Source: CAD feature listing. Evaluate the final solid. Frame: model axes, mm. A direction names the side the tool comes from. Give positions to 0.01 mm unless a question says otherwise; leave off trailing zeros. Loops run counter-clockwise (first coordinate to the right, second up) from the corner with the lowest first, then second, coordinate; pieces in that order, holes last.
from build123d import *

# Parameters (mm, degrees)
BOSS_EXTRUDE1_DEPTH        = 40
SKETCH3_W                  = 100.026130685
SKETCH3_H                  = 60
BOSS_EXTRUDE2_DEPTH        = 25
FILLET1_R                  = 20
F_10_0_10_DIAMETER_HOLE1_D = 10
FILLET1_OF_MIRROR1_R       = 20
DELETEFACE1_START          = -30
DELETEFACE1_DEPTH          = 60
SKETCH16_R                 = 5
BOSS_EXTRUDE3_DEPTH        = 15
RIB1_REACH                 = 138.403
SKETCH18_WALL_W            = 310.161126634
SKETCH18_WALL_H            = 10


# Read off the part's stored shape, not the designer's step: DeleteFace1
with BuildPart() as part:
    # Sketch2 → Boss-Extrude1 (new, symmetric)
    with BuildSketch(Plane.XY):
        with BuildLine():
            Line((-40, 0), (-25, 0))
            ThreePointArc((-25, 0), (0, 25), (25, 0))
            Line((25, 0), (40, 0))
            ThreePointArc((40, 0), (0, 40), (-40, 0))
        make_face()
    extrude(amount=BOSS_EXTRUDE1_DEPTH, both=True)

    # Sketch3 → Boss-Extrude2 (add)
    with BuildSketch(Plane.XZ):
        with Locations((-60.013065343, 0)):
            Rectangle(SKETCH3_W, SKETCH3_H)
    boss_extrude2 = extrude(amount=-BOSS_EXTRUDE2_DEPTH)

    # Fillet1
    fillet1_edges = [part.edges().sort_by_distance(p)[0] for p in [
        (-110.026130685, 12.5, 30),
        (-110.026130685, 12.5, -30),
    ]]
    fillet(fillet1_edges, radius=FILLET1_R)

    # Ø10.0 (10) Diameter Hole1 (through all)
    with Locations(Plane(origin=(0, 25, 0), x_dir=(1, 0, 0), z_dir=(0, 1, 0))):
        with Locations((-90.026130685, -10), (-90.026130685, 11.237902365)):
            f_10_0_10_diameter_hole1 = Hole(F_10_0_10_DIAMETER_HOLE1_D / 2)

    # Mirror1: Boss-Extrude2, Ø10.0 (10) Diameter Hole1 across plane
    add(boss_extrude2.mirror(Plane(origin=(0, 0, 0), x_dir=(0, 0, 1), z_dir=(1, 0, 0))))
    add(f_10_0_10_diameter_hole1.mirror(Plane(origin=(0, 0, 0), x_dir=(0, 0, 1), z_dir=(1, 0, 0))), mode=Mode.SUBTRACT)

    # Fillet1 of Mirror1
    fillet1_of_mirror1_edges = [part.edges().sort_by_distance(p)[0] for p in [
        (110.026130685, 12.5, 30),
        (110.026130685, 12.5, -30),
    ]]
    fillet(fillet1_of_mirror1_edges, radius=FILLET1_OF_MIRROR1_R)

    # DeleteFace1 outline → DeleteFace1 (cut)
    with BuildSketch(Plane.XY.offset(DELETEFACE1_START)):
        with BuildLine():
            ThreePointArc((25, 0), (20.916500663, 13.693063938), (10, 22.912878475))
            Line((10, 22.912878475), (10, 0))
            Line((10, 0), (25, 0))
        make_face()
        with BuildLine():
            ThreePointArc((-10, 22.912878475), (-20.916500663, 13.693063938), (-25, 0))
            Line((-25, 0), (-10, 0))
            Line((-10, 0), (-10, 22.912878475))
        make_face()
    extrude(amount=DELETEFACE1_DEPTH, mode=Mode.SUBTRACT)

    # Sketch16 → Boss-Extrude3 (add, symmetric)
    with BuildSketch(Plane.XY):
        with BuildLine():
            ThreePointArc((20, 34.641016151), (0, 40), (-20, 34.641016151))
            Line((-20, 34.641016151), (-20, 50))
            ThreePointArc((-20, 50), (0, 70), (20, 50))
            Line((20, 50), (20, 34.641016151))
        make_face()
        with Locations((0, 50)):
            Circle(SKETCH16_R, mode=Mode.SUBTRACT)
    extrude(amount=BOSS_EXTRUDE3_DEPTH, both=True)

    # Sketch18 wall → Rib1 (add, up to next)
    with BuildSketch(Plane(origin=(-32.5, 37.5, 0), x_dir=(-0.707106781187, -0.707106781187, 0), z_dir=(0.707106781187, -0.707106781187, 0)), mode=Mode.PRIVATE) as rib1_sk1:
        Rectangle(SKETCH18_WALL_W, SKETCH18_WALL_H)
    rib1_tool1 = extrude(rib1_sk1.sketch, amount=RIB1_REACH, mode=Mode.PRIVATE) - part.part
    rib1 = rib1_tool1.solids().sort_by_distance((-32.5, 37.5, 0))[0]
    add(rib1)

    # Mirror2: Rib1 across plane
    add(rib1.mirror(Plane(origin=(0, 0, 0), x_dir=(0, 0, 1), z_dir=(1, 0, 0))))


solid = part.part
1) Pull-direction query (Y, two-part tool) for faces 1 (the flat face through (71, 25, 0)), 2 (the flat face through (29, 35, 5)), 3 (the cylindrical face through (-0.651, 54.957, -0.21)); classes: released by +Y, released by -Y, zero draft, split by the parting line, or undercut.
Checks:
face 1: released by +Y
face 2: zero draft
face 3: undercut
2) Ray query, probe 1 along Y at (x, z) = (0, -4.25); probe 2 along X at (y, z) = (22.5, -8); probe 3 along X at (y, z) = (17, -9). Return the intervals inside material, ascending.
Checks:
probe 1: y = 25 to 45, 55 to 70
probe 2: x = -110.03 to -93.84, -86.22 to -10.9, 10.9 to 86.22, 93.84 to 110.03
probe 3: x = -110.03 to -94.5, -85.55 to -18.33, 18.33 to 85.55, 94.5 to 110.03
3) Cut plane A-A (x = 0). Return loops of the section in (y, z), and give its area (3 significant figures).
Checks:
outline: (25, -40) - (40, -40) - (40, -15) - (45, -15) - (45, 15) - (40, 15) - (40, 40) - (25, 40) - close; (55, -15) - (70, -15) - (70, 15) - (55, 15) - close
area: 1,800 mm2
4) Contact query for flat-ended pins moving along their axis: P1, Ø9, axis at x = 90.03, z = -11.24, coming from the -Y side; P2, Ø5, axis at x = 52, y = 19.5, coming from the +Z side; P3, Ø1.5, axis at y = 41.5, z = 3.5, coming from the +X side; P4, Ø8, axis at y = 43, z = -10, coming from the +X side. Output: stop coordinate, or through.
Checks:
P1: passes through
P2: stops at z = 30
P3: stops at x = 29.25
P4: stops at x = 20
5) Cut plane B-B (z = -2). Return loops of the section in (x, y), and give its area (3 significant figures).
Checks:
outline: (-110.03, 0) - (-25, 0) arc R25 cw to (25, 0) - (110.03, 0) - (110.03, 25) - (45, 25) - (20, 50) arc R20 ccw to (-20, 50) - (-45, 25) - (-110.03, 25) - close; hole circle Ø10 at (0, 50)
area: 6,690 mm2
6) Reachability of faces 4 (the flat face through (-29, 35, -5)), 5 (the flat face through (29, 35, -5)), 6 (the cylindrical face through (104.32, 12.68, -23.99)), 7 (the flat face through (20, 42, 10)) from +Z, -Z, +X, -X, +Y, -Y: full face, straight path, thin tool, end or side. Return the list, or none.
Checks:
face 4: -Z, -X, +Y
face 5: -Z, +X, +Y
face 6: -Z, +X, +Y, -Y
face 7: +Z, +X, +Y
7) Cut plane D-D (y = 16). Return loops of the section in (x, z), and give its area (3 significant figures).
Checks:
outline: (-110.03, -10) arc R20 ccw to (-90.03, -30) - (-36.66, -30) - (-36.66, -40) - (-19.21, -40) - (-19.21, 40) - (-36.66, 40) - (-36.66, 30) - (-90.03, 30) arc R20 ccw to (-110.03, 10) - close; (19.21, -40) - (36.66, -40) - (36.66, -30) - (90.03, -30) arc R20 ccw to (110.03, -10) - (110.03, 10) arc R20 ccw to (90.03, 30) - (36.66, 30) - (36.66, 40) - (19.21, 40) - close; hole circle Ø10 at (-90.03, -11.24); hole circle Ø10 at (-90.03, 10); hole circle Ø10 at (90.03, -11.24); hole circle Ø10 at (90.03, 10)
area: 10,900 mm2
8) Cut plane C-C (y = 38). Return loops of the section in (x, z).
Checks:
outline: (-32, -5) - (-20, -5) - (-20, -15) - (-12.49, -15) - (-12.49, -40) - (12.49, -40) - (12.49, -15) - (20, -15) - (20, -5) - (32, -5) - (32, 5) - (20, 5) - (20, 15) - (12.49, 15) - (12.49, 40) - (-12.49, 40) - (-12.49, 15) - (-20, 15) - (-20, 5) - (-32, 5) - close
